Here's how the part is built. I have some questions about the finished solid (model axes, mm). Face numbers are marked on the shaded views. Round coordinates to 2 decimals unless told otherwise and drop trailing zeros. Loops run counter-clockwise (first coordinate to the right, second up) from the corner with the lowest first, then second, coordinate; pieces in that order, holes last. Notation, with made-up numbers: M 47.25,54.5 L 73.25,54.5 A20 ccw 73.25,63.5 Z; hole C -31.5,28 d8. An arc over 180 degrees is marked long. Use a Markdown table: item, result.
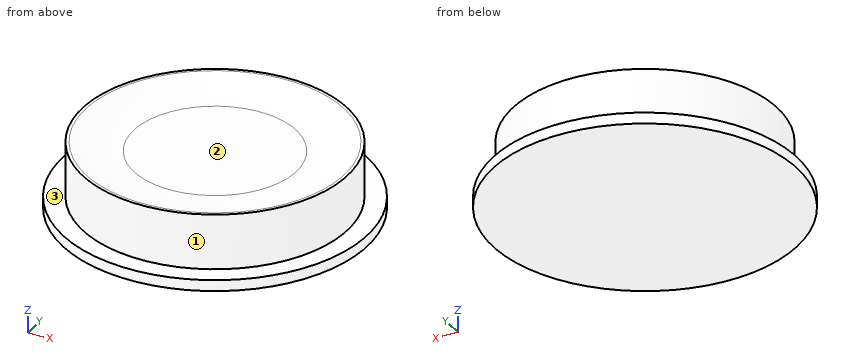
Autodesk Inventor part; units mm, degrees
ref_plane "YZ Plane" through (0, 0, 0) normal (1, 0, 0) x (0, 1, 0)
ref_plane "XZ Plane" through (0, 0, 0) normal (0, 1, 0) x (-1, 0, 0)
ref_plane "XY Plane" through (0, 0, 0) normal (0, 0, 1) x (1, 0, 0)
sketch "Sketch1" plane through (0, 0, 0) normal (0, 0, 1) x (1, 0, 0)
  circle A0 centre (0, 0) radius 7.175
  circle A1 centre (0, 0) radius 8.25
  dimension "d0" = 14.35
  dimension "d1" = 16.5
extrude "Extrusion1" add sketch "Sketch1" along normal blind 3 contours A0
extrude "Extrusion2" add sketch "Sketch1" against normal blind 0.6 contours A0 | A1
sketch "Sketch2" plane through (0, 0, 3) normal (0, 0, 1) x (1, 0, 0)
  circle A0 centre (0, 0) radius 7
  dimension "d6" = 14
extrude "Extrusion3" cut sketch "Sketch2" against normal blind 0.5
fillet "Fillet1" radius 7 1 edges at (-7, 0, 2.5)
properties part number "pwrButton"
Q1. We'd pull the mould along X, two halves only. Please class the marked faces 1, 2 and 3: pulls with the +X half, pulls with the -X half, needs draft (parallel to the pull), parting line crosses it, or undercut.
Return value:
| item | result |
|---|---|
| face 1 | parting line crosses it |
| face 2 | undercut |
| face 3 | needs draft |
Q2. Imagine slicing it at A-A, the plane z = 0.2. Please give me the cut outline in (x, y) (3 decimals), then the cut area to 3 significant figures.
Return value:
| item | result |
|---|---|
| outline | C 0,0 d14.35 |
| area | 162 mm^2 |
Q3. Will these pins go through, and if not, where does the flat tip stop? P1, Ø3, axis at x = -1.5, y = -2, coming from the +Z side; P2, Ø1, axis at y = 6.5, z = 1, coming from the -X side; P3, Ø1.5, axis at x = -5.5, y = 6.5, coming from the +Z side.
Return value:
| item | result |
|---|---|
| P1 | stops at z = 2.5 |
| P2 | stops at x = -3.93 |
| P3 | stops at z = 0 |
Q4. I need wall thicknesses on line 1 (Z direction, x = 3, y = -1.5); line 2 (Z direction, x = -4.5, y = -6.25); line 3 (X direction, y = -1.5, z = -0.15). Which ranges of each line are inside material? Lowest first, please. Write a range as from..to.
Return value:
| item | result |
|---|---|
| line 1 | z = -0.6..2.5 |
| line 2 | z = -0.6..0 |
| line 3 | x = -8.11..8.11 |
